Part model, mm, in its own coordinate system. A direction names the side the tool comes from. Round coordinates to 2 decimals unless told otherwise and drop trailing zeros. Write each loop counter-clockwise with the first axis right and the second up, starting at its lowest first coordinate (ties: lowest second). Pieces come first, ordered by that corner, then holes.
```python
from build123d import *

# Parameters (mm, degrees)
SKETCH1_W           = 24
SKETCH1_H           = 34
SKETCH1_R           = 7.5
BOSS_EXTRUDE1_DEPTH = 28
SKETCH5_W           = 12
SKETCH5_H           = 30
BOSS_EXTRUDE3_DEPTH = 10
SKETCH6_W           = 8
SKETCH6_H           = 5
CUT_EXTRUDE3_DEPTH  = 50.769468553
CUT_EXTRUDE4_REACH  = 55.516
SKETCH7_R           = 1
SKETCH8_R           = 4
CUT_EXTRUDE5_DEPTH  = 20
SKETCH9_W           = 42.3
SKETCH9_H           = 5
BOSS_EXTRUDE4_DEPTH = 42.3
SKETCH10_R          = 12
SKETCH10_R_2        = 1.5
CUT_EXTRUDE6_DEPTH  = 48
FILLET1_R           = 5
FILLET2_R           = 5


with BuildPart() as part:
    # Sketch1 → Boss-Extrude1 (new, symmetric)
    with BuildSketch(Plane.XY):
        with Locations((0, -5)):
            Rectangle(SKETCH1_W, SKETCH1_H)
        Circle(SKETCH1_R, mode=Mode.SUBTRACT)
    extrude(amount=BOSS_EXTRUDE1_DEPTH, both=True)

    # Sketch5 → Boss-Extrude3 (add)
    with BuildSketch(Plane(origin=(0, 12, 0), x_dir=(1, 0, 0), z_dir=(0, 1, 0))):
        with Locations((6, 0)):
            Rectangle(SKETCH5_W, SKETCH5_H)
    extrude(amount=BOSS_EXTRUDE3_DEPTH)

    # Sketch6 → Cut-Extrude3 (cut, through all)
    with BuildSketch(Plane.XY.offset(15)):
        with Locations((4, 14.5)):
            Rectangle(SKETCH6_W, SKETCH6_H)
    extrude(amount=-CUT_EXTRUDE3_DEPTH, mode=Mode.SUBTRACT)

    # Sketch7 → Cut-Extrude4 (cut, up to next)
    with BuildSketch(Plane(origin=(0, 22, 0), x_dir=(1, 0, 0), z_dir=(0, 1, 0)), mode=Mode.PRIVATE) as cut_extrude4_sk1:
        with Locations(Location((4, 11, 0), (0, 0, 270))):
            Circle(SKETCH7_R)
    cut_extrude4_tool1 = extrude(cut_extrude4_sk1.sketch, amount=-CUT_EXTRUDE4_REACH, mode=Mode.PRIVATE) & part.part
    # Sketch7 → Cut-Extrude4 (cut, up to next)
    with BuildSketch(Plane(origin=(0, 22, 0), x_dir=(1, 0, 0), z_dir=(0, 1, 0)), mode=Mode.PRIVATE) as cut_extrude4_sk2:
        with Locations(Location((4, -11, 0), (0, 0, 270))):
            Circle(SKETCH7_R)
    cut_extrude4_tool2 = extrude(cut_extrude4_sk2.sketch, amount=-CUT_EXTRUDE4_REACH, mode=Mode.PRIVATE) & part.part
    add(cut_extrude4_tool1.solids().sort_by_distance((4, 22, -11))[0], mode=Mode.SUBTRACT)
    add(cut_extrude4_tool2.solids().sort_by_distance((4, 22, 11))[0], mode=Mode.SUBTRACT)

    # Sketch8 → Cut-Extrude5 (cut)
    with BuildSketch(Plane(origin=(12, 0, 0), x_dir=(0, 0, -1), z_dir=(1, 0, 0))):
        with Locations(Location((-14, -14, 0), (0, 0, 90))):
            Circle(SKETCH8_R)
        with Locations(Location((14, -14, 0), (0, 0, 90))):
            Circle(SKETCH8_R)
    extrude(amount=-CUT_EXTRUDE5_DEPTH, mode=Mode.SUBTRACT)

    # Sketch9 → Boss-Extrude4 (add)
    with BuildSketch(Plane.XZ.offset(22)):
        with Locations((0, -7.5)):
            Rectangle(SKETCH9_W, SKETCH9_H)
    extrude(amount=BOSS_EXTRUDE4_DEPTH)

    # Sketch10 → Cut-Extrude6 (cut)
    with BuildSketch(Plane(origin=(0, 0, -10), x_dir=(-1, 0, 0), z_dir=(0, 0, -1))):
        with Locations((0, -43.15)):
            Circle(SKETCH10_R)
        with Locations((-15.5, -27.65)):
            Circle(SKETCH10_R_2)
        with Locations((15.5, -27.65)):
            Circle(SKETCH10_R_2)
        with Locations((15.5, -58.65)):
            Circle(SKETCH10_R_2)
        with Locations((-15.5, -58.65)):
            Circle(SKETCH10_R_2)
    extrude(amount=-CUT_EXTRUDE6_DEPTH, mode=Mode.SUBTRACT)

    # Fillet1
    fillet1_edges = [part.edges().sort_by_distance(p)[0] for p in [
        (-12, -22, -7.5),
    ]]
    fillet(fillet1_edges, radius=FILLET1_R)

    # Fillet2
    fillet2_edges = [part.edges().sort_by_distance(p)[0] for p in [
        (12, -22, -7.5),
    ]]
    fillet(fillet2_edges, radius=FILLET2_R)


solid = part.part
```
Q1. Which spindle directions (+Z, -Z, +X, -X, +Y, -Y) get a long thin tool onto all of the face, cutting with end or side? Do faces 1 (the flat face through (-19, -22, -7)), 2 (the flat face through (7, 18, -15)), 3 (the flat face through (8, 14, 0)), 4 (the cylindrical face through (2, -18, 14)), 5 (the cylindrical face through (4.676, 19.535, 10.263)). Say none if no direction does.
Values follow:
face 1: +Z, -Z, -X, +Y
face 2: -Z, +X, -X, +Y
face 3: +Z, -Z, -X
face 4: +X
face 5: +Y
Q2. Cut at A-A on y = -43.15. Write the cut outline in (x, z), plus the area to 3 significant figures.
Values follow:
outline: (-21.15, -10) - (-12, -10) - (-12, -5) - (-21.15, -5) - close; (12, -10) - (21.15, -10) - (21.15, -5) - (12, -5) - close
area: 91.5 mm2
Q3. Wall check: L1, parallel to Z at x = 0.75, y = -14; L2, parallel to X at y = -60, z = -7.5; L3, parallel to Y at x = 15.5, z = -8.25. Give the ranges that are in metal, low to high.
Values follow:
L1: z = -28 to -18, -10 to 10, 18 to 28
L2: x = -21.15 to -16.15, -14.85 to 14.85, 16.15 to 21.15
L3: y = -64.3 to -60.15, -57.15 to -29.15, -26.15 to -21.77
Q4. Cut at C-C on z = 14. Write the cut outline in (x, y).
Values follow:
outline: (-12, -22) - (12, -22) - (12, -18) - (-8, -18) - (-8, -10) - (12, -10) - (12, 22) - (0, 22) - (0, 17) - (8, 17) - (8, 12) - (-12, 12) - close; hole circle Ø15 at (0, 0)
Q5. Mould opens along Y. For faces 6 (the cylindrical face through (-14.39, -57.64, -7.54)), 7 (the flat face through (0, -22, -19)), 8 (the cylindrical face through (-14, -21, -7)) say: +Y half, -Y half, draft (parallel to the pull), parting line (faces both ways), or undercut.
Values follow:
face 6: undercut
face 7: -Y half
face 8: +Y half
Q6. Cut at B-B on x = 4. State how many separate pieces and enclosed holes the cut face has, plus the area to 3 significant figures.
Values follow:
separate pieces: 6
enclosed holes: 2
area: 1,320 mm2
Q7. Drop flat-ended pins along their axis: pin 1 (2 mm diameter, centred on y = -3, z = -4, fed in from +X); pin 2 (5.5 mm diameter, centred on y = 20, z = -6, fed in from -X); pin 3 (5 mm diameter, centred on x = -9.5, z = 13, fed in from +Y); pin 4 (14.5 mm diameter, centred on x = 0, y = -43.15, fed in from +Z). Give the stop position or say it passes through.
Values follow:
pin 1: stops at x = 12
pin 2: stops at x = 0
pin 3: stops at y = 12
pin 4: passes through
Q8. Cut at D-D on z = -8. Write the cut outline in (x, y).
Values follow:
outline: (-21.15, -64.3) - (21.15, -64.3) - (21.15, -22) - (17, -22) arc R5 cw to (12, -17) - (12, 22) - (0, 22) - (0, 17) - (8, 17) - (8, 12) - (-12, 12) - (-12, -17) arc R5 cw to (-17, -22) - (-21.15, -22) - close; hole circle Ø3 at (-15.5, -58.65); hole circle Ø3 at (-15.5, -27.65); hole circle Ø24 at (0, -43.15); hole circle Ø15 at (0, 0); hole circle Ø3 at (15.5, -58.65); hole circle Ø3 at (15.5, -27.65)
